Here's how the part is built. I have some questions about the finished solid (model axes, mm). Face numbers are marked on the shaded views. A direction names the side the tool comes from. Coordinates: 2 decimals unless noted, no trailing zeros. Order: outer loops, then holes, each group sorted by start corner. A loop starts at its lowest first (then second) coordinate and runs counter-clockwise, first axis right, second up. Notation, with made-up numbers: M 31,46 L 80,46 A9 cw 80,61 Z; hole C 63,13.5 d5. An arc over 180 degrees is marked long. Answer as CSV lines item,"result". Start each with the question number.
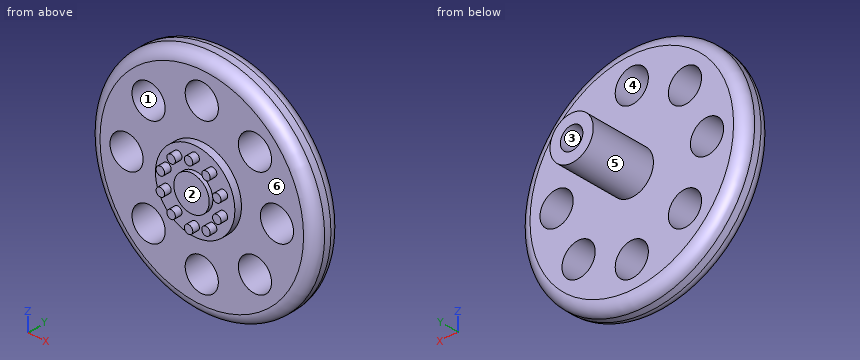
```python
from build123d import *

# Parameters (mm, degrees)
F0_R      = 15.621
F1_DEPTH  = 4
F2_R      = 2.4511
F3_DEPTH  = 1.55
F4_R      = 2.9972
F5_DEPTH  = 9.1
F6_R      = 1.555
F7_DEPTH  = 6
F9_R      = 5.5
F10_DEPTH = 1
F11_R     = 1.524
F12_R     = 1.524
F13_R     = 0.58563
F14_DEPTH = 1
F15_R     = 2.297006
F16_DEPTH = 25.4


with BuildPart() as f1:
    # F0 (on Front) → F1 (new body)
    with BuildSketch(Plane.XZ):
        Circle(F0_R)
    extrude(amount=F1_DEPTH)

    # F2 (on face) → F3 (join)
    with BuildSketch(Plane.XZ.offset(4)):
        Circle(F2_R)
    extrude(amount=F3_DEPTH)

    # F4 (on face) → F5 (join)
    with BuildSketch(Plane.XZ):
        Circle(F4_R)
    extrude(amount=-F5_DEPTH)

    # F6 (on face) → F7 (cut)
    with BuildSketch(Plane(origin=(0, 9.1, 0), x_dir=(-1, 0, 0), z_dir=(0, 1, 0))):
        Circle(F6_R)
    extrude(amount=-F7_DEPTH, mode=Mode.SUBTRACT)

    # F9 (on face) → F10 (join)
    with BuildSketch(Plane.XZ.offset(4)):
        Circle(F9_R)
    extrude(amount=F10_DEPTH)

    # F11
    f11_edges = [f1.edges().sort_by_distance(p)[0] for p in [
        (-15.621, -4, 0),
    ]]
    fillet(f11_edges, radius=F11_R)

    # F12
    f12_edges = [f1.edges().sort_by_distance(p)[0] for p in [
        (-15.621, 0, 0),
    ]]
    fillet(f12_edges, radius=F12_R)

    # F13 (on face) → F14 (join)
    with BuildSketch(Plane.XZ.offset(5)):
        with Locations((3.908391, -1.269913)):
            Circle(F13_R)
        with Locations((0, -4.109526)):
            Circle(F13_R)
        with Locations((-3.908391, -1.269913)):
            Circle(F13_R)
        with Locations((-2.415519, -3.324676)):
            Circle(F13_R)
        with Locations((-3.908391, 1.269913)):
            Circle(F13_R)
        with Locations((-2.415519, 3.324676)):
            Circle(F13_R)
        with Locations((0, 4.109526)):
            Circle(F13_R)
        with Locations((2.415519, 3.324676)):
            Circle(F13_R)
        with Locations((3.908391, 1.269913)):
            Circle(F13_R)
        with Locations((2.415519, -3.324676)):
            Circle(F13_R)
    extrude(amount=F14_DEPTH)

    # F15 (on face) → F16 (cut)
    with BuildSketch(Plane.XZ.offset(4)):
        with Locations((7.366795, 7.366795)):
            Circle(F15_R)
        with Locations((0, 10.418221)):
            Circle(F15_R)
        with Locations((-7.366795, 7.366795)):
            Circle(F15_R)
        with Locations((-10.418221, 0)):
            Circle(F15_R)
        with Locations((-7.366795, -7.366795)):
            Circle(F15_R)
        with Locations((0, -10.418221)):
            Circle(F15_R)
        with Locations((7.366795, -7.366795)):
            Circle(F15_R)
        with Locations((10.418221, 0)):
            Circle(F15_R)
    extrude(amount=-F16_DEPTH, mode=Mode.SUBTRACT)


solid = f1.part
```
1) I need wall thicknesses on line 1 (Z direction, x = 0, y = -1.7); line 2 (Z direction, x = 6, y = -2.25); line 3 (Y direction, x = -10.5, z = -9.5). Which ranges of each line are inside material? Lowest first, please. Write a range as [from, to].
2) Suppose I cut it at A-A on z = 0. Give the number of separate pieces and of enclosed holes in the cut face, plus the area to 3 significant figures.
3) Will these pins go through, and if not, where does the flat tip stop? pin 1 Ø2.5 at (x, z) = (0, 0) entering from +Y; pin 2 Ø12 at (x, z) = (5.5, -10) entering from -Y; pin 3 Ø2.5 at (x, z) = (0, 0) entering from -Y; pin 4 Ø3.5 at (x, z) = (0, 10.42) entering from +Y.
4) If we mould it in two halves opening along Z, with no side actions, what happens to the marked faces 4, 5 and 6? For each: released by +Z, released by -Z, zero draft, split by the parting line, or undercut.
5) Suppose I cut it at D-D on y = 1. Please give me the cut outline in (x, z), plus the area to 3 significant figures.
6) Which directions (+Z, -Z, +X, -X, +Y, -Y) give clear straight access to the entire face, cutting with the end or side of a thin tool? Please do the marked faces 1, 2 and 3.
Output:
1,line 1,"[-15.62, -12.72], [-8.12, 8.12], [12.72, 15.62]"
1,line 2,"[-14.42, -9.21], [-5.52, 5.52], [9.21, 14.42]"
1,line 3,"[-4, 0]"
2,separate pieces,"3"
2,enclosed holes,"0"
2,area,"136 mm²"
3,pin 1,"y = 3.1"
3,pin 2,"y = -5"
3,pin 3,"y = -5.55"
3,pin 4,"through"
4,face 4,"undercut"
4,face 5,"split by the parting line"
4,face 6,"zero draft"
5,outline,"C 0,0 d5.99"
5,area,"28.2 mm²"
6,face 1,"+Y, -Y"
6,face 2,"-Y"
6,face 3,"+Y"
